Input: part model. Units: mm. Frame: model coordinates. A direction names the side the tool comes from. Round coordinates to 2 decimals unless told otherwise and drop trailing zeros. Order: outer loops, then holes, each group sorted by start corner. A loop starts at its lowest first (then second) coordinate and runs counter-clockwise, first axis right, second up.
Item 1: Cut plane B-B on x = 1. Output: boundary loops of the cut face in (y, z).
Item 2: Reachability of faces 4 (the flat face through (-6.972, 2, 0)), 5 (the flat face through (0, -1, 6.35)), 6 (the flat face through (0, 2, 6.972)) from +Z, -Z, +X, -X, +Y, -Y: full face, straight path, thin tool, end or side. Return the list, or none.
Item 3: Mould query, pull axis Y, two halves, no side actions, for faces 1 (the flat face through (0, 2, -6.972)), 2 (the flat face through (0, -2.413, 0)), 3 (the flat face through (0, 1, 6.21)). Classes: released by +Y, released by -Y, zero draft, split by the parting line, or undercut.
Item 4: Cut plane A-A on z = 4.25. Output: boundary loops of the cut face in (x, y), then the cut area to 3 significant figures.
Item 5: Cut plane C-C on y = 1.25. Output: boundary loops of the cut face in (x, z), then the cut area to 3 significant figures.
Item 6: Line query: L1, parallel to X at y = -0.75, z = -1.5; L2, parallel to Z at x = -4.5, y = 1.75. Output: solid intervals per line, ascending.
Item 7: First-contact query: pin 1 (0.8 mm diameter, centred on y = 1, z = 6.5, fed in from -X); pin 2 (1.9 mm diameter, centred on x = 1.5, y = -1.5, fed in from -Z); pin 3 (2 mm diameter, centred on x = 3, y = 1.5, fed in from +Z). Flat tips, straight axial feed; report the tip coordinate or a pass-through.
Item 8: Cut plane D-D on x = -2.75. Output: boundary loops of the cut face in (y, z), then the cut area to 3 significant figures.
Autodesk Inventor part; units mm, degrees
ref_plane "diffuser_to_body_XY" through (0, 0, 0) normal (0, 1, 0) x (1, 0, 0)
ref_plane "diffuser_to_body_YZ" through (0, 0, 0) normal (1, 0, 0) x (0, 0, -1)
ref_plane "diffuser_to_body_ZX" through (0, 0, 0) normal (0, 0, -1) x (0, 1, 0)
sketch "Sketch_1" plane through (0, 0, 0) normal (0, 1, 0) x (-1, 0, 0)
  line L0 (7.5057, 7.5057) -> (-7.5057, 7.5057)
  line L1 (-7.5057, 7.5057) -> (-7.5057, -7.5057)
  line L2 (-7.5057, -7.5057) -> (7.5057, -7.5057)
  line L3 (7.5057, -7.5057) -> (7.5057, 7.5057)
extrude "Extrusion1" add sketch "Sketch_1" along normal blind 4.0894
sketch "Sketch_2" plane through (0, 0.254, 0) normal (0, 1, 0) x (1, 0, 0)
  line L0 (-7.62, -7.62) -> (7.62, -7.62)
  line L1 (7.62, -7.62) -> (7.62, 7.62)
  line L2 (7.62, 7.62) -> (-7.62, 7.62)
  line L3 (-7.62, 7.62) -> (-7.62, -7.62)
  line L4 (-6.9723, -6.9723) -> (6.9723, -6.9723)
  line L5 (6.9723, -6.9723) -> (6.9723, 6.9723)
  line L6 (6.9723, 6.9723) -> (-6.9723, 6.9723)
  line L7 (-6.9723, 6.9723) -> (-6.9723, -6.9723)
extrude "Extrusion2" cut sketch "Sketch_2" along normal blind 6.35
sketch "Sketch_4" plane through (0, 0, 6.9723) normal (0, 0, 1) x (1, 0, 0)
  line L0 (-1.778, 0.254) -> (1.778, 0.254)
  line L1 (1.778, 0.254) -> (1.778, 1.524)
  line L2 (1.778, 1.524) -> (-1.778, 1.524)
  line L3 (-1.778, 1.524) -> (-1.778, 0.254)
extrude "Extrusion3" cut sketch "Sketch_4" against normal blind 0.762
sketch "Sketch_6" plane through (0, 0, 0) normal (0, 1, 0) x (-1, 0, 0)
  line L0 (6.35, 6.35) -> (-6.35, 6.35)
  line L1 (-6.35, 6.35) -> (-6.35, -6.35)
  line L2 (-6.35, -6.35) -> (6.35, -6.35)
  line L3 (6.35, -6.35) -> (6.35, 6.35)
extrude "Extrusion4" add sketch "Sketch_6" against normal blind 2.413
ref_plane "diffuser_to_body_XY" through (0, 0, 0) normal (0, 1, 0) x (1, 0, 0)
ref_plane "diffuser_to_body_YZ" through (0, 0, 0) normal (1, 0, 0) x (0, 0, -1)
ref_plane "diffuser_to_body_ZX" through (0, 0, 0) normal (0, 0, -1) x (0, 1, 0)
ref_plane "diffuser_to_body_green_XY" through (3.7529, 0, 0) normal (0, 1, 0) x (1, 0, 0)
ref_plane "diffuser_to_body_green_YZ" through (3.7529, 0, 0) normal (1, 0, 0) x (0, 0, -1)
ref_plane "diffuser_to_body_green_ZX" through (3.7529, 0, 0) normal (0, 0, -1) x (0, 1, 0)
ref_plane "diffuser_to_body_red_XY" through (-3.7529, 0, 0) normal (0, 1, 0) x (1, 0, 0)
ref_plane "diffuser_to_body_red_YZ" through (-3.7529, 0, 0) normal (1, 0, 0) x (0, 0, -1)
ref_plane "diffuser_to_body_red_ZX" through (-3.7529, 0, 0) normal (0, 0, -1) x (0, 1, 0)
properties part number "UB216SKG035D-1JBd_cap"
From the geometry:
1. outline: (-2.41, -6.35) - (0, -6.35) - (0, -7.51) - (0.25, -7.51) - (0.25, -6.97) - (4.09, -6.97) - (4.09, 6.97) - (1.52, 6.97) - (1.52, 6.21) - (0.25, 6.21) - (0.25, 7.51) - (0, 7.51) - (0, 6.35) - (-2.41, 6.35) - close
2. face 4: +Z, -Z, -X, +Y
2. face 5: +Z, +X, -X, -Y
2. face 6: +Z, +X, -X, +Y
3. face 1: zero draft
3. face 2: released by -Y
3. face 3: undercut
4. outline: (-7.51, 0) - (-6.35, 0) - (-6.35, -2.41) - (6.35, -2.41) - (6.35, 0) - (7.51, 0) - (7.51, 0.25) - (6.97, 0.25) - (6.97, 4.09) - (-6.97, 4.09) - (-6.97, 0.25) - (-7.51, 0.25) - close
4. area: 87.9 mm2
5. outline: (-6.97, -6.97) - (6.97, -6.97) - (6.97, 6.97) - (1.78, 6.97) - (1.78, 6.21) - (-1.78, 6.21) - (-1.78, 6.97) - (-6.97, 6.97) - close
5. area: 192 mm2
6. L1: x = -6.35 to 6.35
6. L2: z = -6.97 to 6.97
7. pin 1: stops at x = -6.97
7. pin 2: stops at z = -6.35
7. pin 3: stops at z = 6.97
8. outline: (-2.41, -6.35) - (0, -6.35) - (0, -7.51) - (0.25, -7.51) - (0.25, -6.97) - (4.09, -6.97) - (4.09, 6.97) - (0.25, 6.97) - (0.25, 7.51) - (0, 7.51) - (0, 6.35) - (-2.41, 6.35) - close
8. area: 87.9 mm2
